Geometry: final body of the model. Coordinates: model frame, mm. A direction names the side the tool comes from. Round coordinates to 2 decimals unless told otherwise and drop trailing zeros. Loops run counter-clockwise (first coordinate to the right, second up) from the corner with the lowest first, then second, coordinate; pieces in that order, holes last. Notation, with made-up numbers: (-17, 5.25) - (34, 5.25) arc R29 ccw to (34, 37.25) - close; hole circle Ø7 at (-33.5, 0.25). An arc over 180 degrees is marked (long way). Write item = value, one per line. Start each with the question number.
Item 1: Line query: line 1 (Z direction, x = -75, y = -3.5); line 2 (Y direction, x = -199, z = -145.5); line 3 (X direction, y = -1.5, z = -128). Output: solid intervals per line, ascending. Write a range as from..to.
Item 2: Section A-A (z = -148.5). Return loops of the section in (x, y).
Item 3: Access query for faces 1 (the flat face through (-104, 4, -146)), 2 (the cylindrical face through (-25.406, -2.028, -188.719)), 3 (the cylindrical face through (-184.594, -2.028, -108.281)), 4 (the cylindrical face through (-184.719, -2.028, -188.594)), 5 (the cylindrical face through (-25.281, -2.028, -108.406)). Directions: +Z, -Z, +X, -X, +Y, -Y. A direction counts if a zero-diameter tool reaches every point of the face in a straight line with its end or side. Return the directions, or none.
Item 4: Section C-C (z = -226.5). Return loops of the section in (x, y).
Item 5: First-contact query: pin 1 (3 mm diameter, centred on y = -2.5, z = -155.5, fed in from -X); pin 2 (1.2 mm diameter, centred on x = -92.5, y = -2, fed in from +Z); pin 3 (6 mm diameter, centred on x = -47.5, z = -55, fed in from -Y). Flat tips, straight axial feed; report the tip coordinate or a pass-through.
Item 6: Section B-B (x = -117.5). Return loops of the section in (y, z).
Autodesk Inventor part; units mm, degrees
ref_plane "YZ Plane" through (0, 0, 0) normal (1, 0, 0) x (0, 1, 0)
ref_plane "XZ Plane" through (0, 0, 0) normal (0, 1, 0) x (-1, 0, 0)
ref_plane "XY Plane" through (0, 0, 0) normal (0, 0, 1) x (1, 0, 0)
sketch "Sketch1" plane through (0, 0, 0) normal (0, 1, 0) x (-1, 0, 0)
  line L0 (0, 0) -> (210, 0)
  line L1 (210, 0) -> (210, -297)
  line L2 (210, -297) -> (0, -297)
  line L3 (0, -297) -> (0, 0)
  line L4 (23, -106) -> (187, -106)
  line L5 (187, -106) -> (187, -191)
  line L6 (187, -191) -> (23, -191)
  line L7 (23, -191) -> (23, -106)
  dimension "d30" = 210
  dimension "d31" = 297
  dimension "d34" = 164
  dimension "d35" = 85
  dimension "d42" = 106
  dimension "d43" = 23
extrude "Extrusion6" add sketch "Sketch1" against normal blind 4 contours L4 L5 L6 L7
extrude "Extrusion7" add sketch "Sketch1" along normal blind 4 contours L0 L1 L2 L3 | L4 L5 L6 L7
fillet "Fillet3" radius 2 4 edges at (0, 2, 0) (-210, 2, 0) (-210, 2, -297) (0, 2, -297)
fillet "Fillet4" radius 8 4 edges at (-187, -2, -191) (-187, -2, -106) (-23, -2, -106) (-23, -2, -191)
sketch "Sketch3" plane through (0, 4, 0) normal (0, 1, 0) x (1, 0, 0)
  line L0 (-210, 295) -> (-210, 2)
  line L1 (-210, 148.5) -> (0, 148.5)
  line L2 (0, 2) -> (0, 295)
  line L3 (-208, 0) -> (-2, 0)
  line L4 (-105, 0) -> (-105, 297)
  line L5 (-2, 297) -> (-208, 297)
  point P0 (0, 0)
Taken from the geometry:
q1.line_1 = -191..-106
q1.line_2 = 0..4
q1.line_3 = -187..-23
q2.outline = (-210, 0) - (-187, 0) - (-187, -4) - (-23, -4) - (-23, 0) - (0, 0) - (0, 4) - (-210, 4) - close
q3.face_1 = +Z, -Z, +X, -X, +Y
q3.face_2 = -Z, +X, -Y
q3.face_3 = +Z, -X, -Y
q3.face_4 = -Z, -X, -Y
q3.face_5 = +Z, +X, -Y
q4.outline = (-210, 0) - (0, 0) - (0, 4) - (-210, 4) - close
q5.pin_1 = -187
q5.pin_2 = -106
q5.pin_3 = 0
q6.outline = (-4, -191) - (0, -191) - (0, -297) - (4, -297) - (4, 0) - (0, 0) - (0, -106) - (-4, -106) - close
